Design review of the part built by this model. Coordinates are the model's own, in mm. Face numbers are marked on the shaded views. A direction names the side the tool comes from. Round coordinates to 2 decimals unless told otherwise and drop trailing zeros. Loops run counter-clockwise (first coordinate to the right, second up) from the corner with the lowest first, then second, coordinate; pieces in that order, holes last. Notation, with made-up numbers: (-26.5, 67) - (17.5, 67) arc R17 ccw to (17.5, 99) - close; hole circle Ø5 at (-11, 53.25). An arc over 180 degrees is marked (long way). Use one line per item in the form item = value. Start each with the question number.
(1) For pin 1 (1.5 mm diameter, centred on x = -24.5, z = 41.5, fed in from -Y); pin 2 (1 mm diameter, centred on x = 54, z = -42.5, fed in from +Y); pin 3 (8 mm diameter, centred on x = 16.5, y = 124, fed in from -Z); pin 4 (21 mm diameter, centred on x = 3.5, z = 10, fed in from -Y), all flat-tipped, find the tip position at first contact; note any pin that passes through.
(2) We need section D-D, the plane z = -61. Write out the cut boundary in (x, y).
(3) Machinability: for the marked faces 1 and 2, which of the approach directions +Z, -Z, +X, -X, +Y, -Y give a long, thin tool a straight path to every point of the face, cutting with its end or side? Answer none if there is none.
(4) We need section A-A, the plane x = 0. Write out the cut boundary in (y, z), then the cut area to 3 significant figures.
(5) We need section B-B, the plane z = 0. Write out the cut boundary in (x, y).
(6) Wall thickness on probe 1 along X at (y, z) = (1.05, 0); probe 2 along X at (y, z) = (148, 0): over which ranges is each line inside the solid? List them lowest first. Write a range as [from, to].
(7) The part is to be moulded in two halves that separate along X. For the marked faces 3, 4 and 5, say which applies: released by +X, released by -X, zero draft, split by the parting line, or undercut.
(8) We need section C-C, the plane y = 42.5. Write out the cut boundary in (x, z), then the cut area to 3 significant figures.
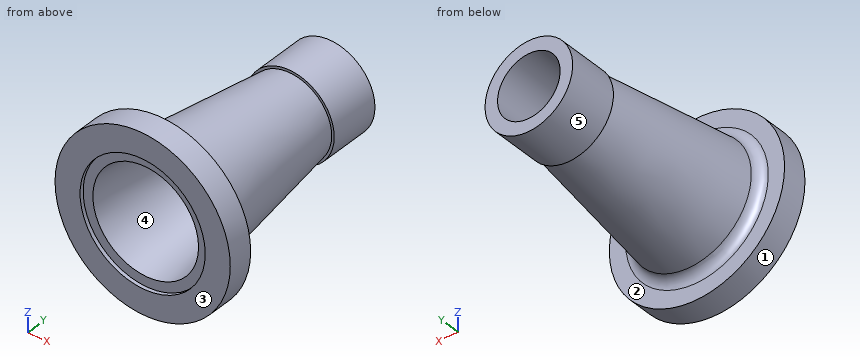
from build123d import *

# Parameters (mm, degrees)
FILLET1_R = 8


with BuildPart() as part:
    # Sketch1 → Revolve1 (revolve)
    with BuildSketch(Plane.XY):
        Polygon((50, 0), (70, 0), (70, 20), (50, 20), (33, 145), (35, 145), (35, 185), (25, 185), (25, 129.61723322), (42.219943718, 3), (50, 3), align=None)
    revolve(axis=Axis((0, 0, 0), (0, 1, 0)))

    # Fillet1
    fillet1_edges = [part.edges().sort_by_distance(p)[0] for p in [
        (-50, 20, 0),
    ]]
    fillet(fillet1_edges, radius=FILLET1_R)


solid = part.part
Data:
q1.pin_1 = 3
q1.pin_2 = 20
q1.pin_3 = -33.72
q1.pin_4 = through
q2.outline = (-34.34, 0) - (34.34, 0) - (34.34, 20) - (-34.34, 20) - close
q3.face_1 = +Y, -Y
q3.face_2 = +Y
q4.outline = (0, -70) - (20, -70) - (20, -56.99) arc R8 cw to (26.92, -49.06) - (145, -33) - (145, -35) - (185, -35) - (185, -25) - (129.62, -25) - (3, -42.22) - (3, -50) - (0, -50) - close; (0, 50) - (3, 50) - (3, 42.22) - (129.62, 25) - (185, 25) - (185, 35) - (145, 35) - (145, 33) - (26.92, 49.06) arc R8 cw to (20, 56.99) - (20, 70) - (0, 70) - close
q4.area = 4,410 mm^2
q5.outline = (-70, 0) - (-50, 0) - (-50, 3) - (-42.22, 3) - (-25, 129.62) - (-25, 185) - (-35, 185) - (-35, 145) - (-33, 145) - (-49.06, 26.92) arc R8 cw to (-56.99, 20) - (-70, 20) - close; (25, 129.62) - (42.22, 3) - (50, 3) - (50, 0) - (70, 0) - (70, 20) - (56.99, 20) arc R8 cw to (49.06, 26.92) - (33, 145) - (35, 145) - (35, 185) - (25, 185) - close
q6.probe_1 = [-70, -50], [50, 70]
q6.probe_2 = [-35, -25], [25, 35]
q7.face_3 = zero draft
q7.face_4 = undercut
q7.face_5 = split by the parting line
q8.outline = circle Ø93.88 at (0, 0); hole circle Ø73.7 at (0, 0)
q8.area = 2,660 mm^2
